Work out the finished part from the listing and answer in its coordinate system (mm). Coordinates: 2 decimals unless noted, no trailing zeros. Loops run counter-clockwise (first coordinate to the right, second up) from the corner with the lowest first, then second, coordinate; pieces in that order, holes last.
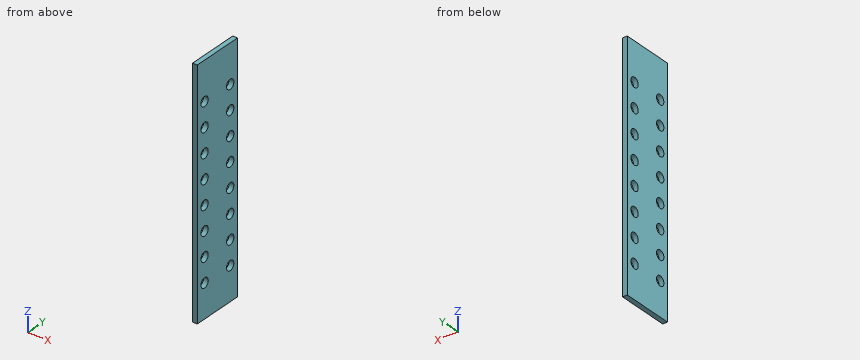
```python
from build123d import *

# Parameters (mm, degrees)
SKETCH2_W               = 500
SKETCH2_H               = 150
BOSS_EXTRUDE1_DEPTH     = 10
SKETCH3_R               = 10
CUT_EXTRUDE1_DEPTH      = 10
LPATTERN1_COUNT         = 8
LPATTERN1_PITCH         = 50
MIRROR1_COPY_1_SKETCH_R = 10
MIRROR1_COPY_1_DEPTH    = 10
MIRROR1_COPY_2_SKETCH_R = 10
MIRROR1_COPY_2_DEPTH    = 10
MIRROR1_COPY_3_SKETCH_R = 10
MIRROR1_COPY_3_DEPTH    = 10
MIRROR1_COPY_4_SKETCH_R = 10
MIRROR1_COPY_4_DEPTH    = 10
MIRROR1_COPY_5_SKETCH_R = 10
MIRROR1_COPY_5_DEPTH    = 10
MIRROR1_COPY_6_SKETCH_R = 10
MIRROR1_COPY_6_DEPTH    = 10
MIRROR1_COPY_7_SKETCH_R = 10
MIRROR1_COPY_7_DEPTH    = 10
SKETCH4_W               = 500
SKETCH4_H               = 19.989679831
SKETCH4_H_2             = 19.964210349
CUT_EXTRUDE2_DEPTH      = 10


with BuildPart() as part:
    # Sketch2 → Boss-Extrude1 (new body)
    with BuildSketch(Plane(origin=(0, 0, 0), x_dir=(0, 0, -1), z_dir=(1, 0, 0))):
        with Locations((250, 75)):
            Rectangle(SKETCH2_W, SKETCH2_H)
    extrude(amount=BOSS_EXTRUDE1_DEPTH)

    # Sketch3 → Cut-Extrude1 (cut)
    with BuildSketch(Plane(origin=(10, 0, 0), x_dir=(0, 0, -1), z_dir=(1, 0, 0))):
        with Locations((80, 110)):
            Circle(SKETCH3_R)
    cut_extrude1 = extrude(amount=-CUT_EXTRUDE1_DEPTH, mode=Mode.SUBTRACT)

    # LPattern1: Cut-Extrude1 ×8
    with Locations(*[(0, 0, -i * LPATTERN1_PITCH) for i in range(1, LPATTERN1_COUNT)]):
        add(cut_extrude1, mode=Mode.SUBTRACT)

    # Mirror1: Cut-Extrude1 across plane
    add(cut_extrude1.mirror(Plane.ZX.offset(75)), mode=Mode.SUBTRACT)

    # Mirror1 copy 1 sketch → Mirror1 copy 1 (cut)
    with BuildSketch(Plane(origin=(10, 150, -50), x_dir=(0, 0, -1), z_dir=(1, 0, 0))):
        with Locations((80, -110)):
            Circle(MIRROR1_COPY_1_SKETCH_R)
    extrude(amount=-MIRROR1_COPY_1_DEPTH, mode=Mode.SUBTRACT)

    # Mirror1 copy 2 sketch → Mirror1 copy 2 (cut)
    with BuildSketch(Plane(origin=(10, 150, -100), x_dir=(0, 0, -1), z_dir=(1, 0, 0))):
        with Locations((80, -110)):
            Circle(MIRROR1_COPY_2_SKETCH_R)
    extrude(amount=-MIRROR1_COPY_2_DEPTH, mode=Mode.SUBTRACT)

    # Mirror1 copy 3 sketch → Mirror1 copy 3 (cut)
    with BuildSketch(Plane(origin=(10, 150, -150), x_dir=(0, 0, -1), z_dir=(1, 0, 0))):
        with Locations((80, -110)):
            Circle(MIRROR1_COPY_3_SKETCH_R)
    extrude(amount=-MIRROR1_COPY_3_DEPTH, mode=Mode.SUBTRACT)

    # Mirror1 copy 4 sketch → Mirror1 copy 4 (cut)
    with BuildSketch(Plane(origin=(10, 150, -200), x_dir=(0, 0, -1), z_dir=(1, 0, 0))):
        with Locations((80, -110)):
            Circle(MIRROR1_COPY_4_SKETCH_R)
    extrude(amount=-MIRROR1_COPY_4_DEPTH, mode=Mode.SUBTRACT)

    # Mirror1 copy 5 sketch → Mirror1 copy 5 (cut)
    with BuildSketch(Plane(origin=(10, 150, -250), x_dir=(0, 0, -1), z_dir=(1, 0, 0))):
        with Locations((80, -110)):
            Circle(MIRROR1_COPY_5_SKETCH_R)
    extrude(amount=-MIRROR1_COPY_5_DEPTH, mode=Mode.SUBTRACT)

    # Mirror1 copy 6 sketch → Mirror1 copy 6 (cut)
    with BuildSketch(Plane(origin=(10, 150, -300), x_dir=(0, 0, -1), z_dir=(1, 0, 0))):
        with Locations((80, -110)):
            Circle(MIRROR1_COPY_6_SKETCH_R)
    extrude(amount=-MIRROR1_COPY_6_DEPTH, mode=Mode.SUBTRACT)

    # Mirror1 copy 7 sketch → Mirror1 copy 7 (cut)
    with BuildSketch(Plane(origin=(10, 150, -350), x_dir=(0, 0, -1), z_dir=(1, 0, 0))):
        with Locations((80, -110)):
            Circle(MIRROR1_COPY_7_SKETCH_R)
    extrude(amount=-MIRROR1_COPY_7_DEPTH, mode=Mode.SUBTRACT)

    # Sketch4 → Cut-Extrude2 (cut)
    with BuildSketch(Plane.ZY):
        with Locations((-250, 140.005160085)):
            Rectangle(SKETCH4_W, SKETCH4_H)
        with Locations((-250, 9.982105175)):
            Rectangle(SKETCH4_W, SKETCH4_H_2)
    extrude(amount=-CUT_EXTRUDE2_DEPTH, mode=Mode.SUBTRACT)


solid = part.part
```
1. Straight lines are drawn through the part: probe 1 along Y at (x, z) = (6, -380); probe 2 along Y at (x, z) = (0.75, -374.5). For each, find the intervals that lie inside material, in ascending order.
2. A cutting plane is placed at A-A, the plane x = 7.5. Count the separate pieces of the cut face and the enclosed holes in it, then the cut area to 3 significant figures.
3. A cutting plane is placed at D-D, the plane z = -230.5. Give the vertices of the cut face in (x, y).
4. A cutting plane is placed at B-B, the plane z = -130. Give the vertices of the cut face in (x, y).
Answers below:
1. probe 1: y = 19.96 to 30, 50 to 100, 120 to 130.01
1. probe 2: y = 19.96 to 31.65, 48.35 to 101.65, 118.35 to 130.01
2. separate pieces: 1
2. enclosed holes: 16
2. area: 50,000 mm2
3. outline: (0, 19.96) - (10, 19.96) - (10, 30.01) - (0, 30.01) - close; (0, 49.99) - (10, 49.99) - (10, 100.01) - (0, 100.01) - close; (0, 119.99) - (10, 119.99) - (10, 130.01) - (0, 130.01) - close
4. outline: (0, 19.96) - (10, 19.96) - (10, 30) - (0, 30) - close; (0, 50) - (10, 50) - (10, 100) - (0, 100) - close; (0, 120) - (10, 120) - (10, 130.01) - (0, 130.01) - close
